from build123d import *

# Parameters (mm, degrees)
BOSS_EXTRU_1_DEPTH = 6


with BuildPart() as part:
    # Esquisse1 → Boss.-Extru.1 (new body)
    with BuildSketch(Plane.XY):
        with BuildLine():
            Line((-20.173501956, 71.960204906), (0, 185.65))
            Line((0, 185.65), (26, 157.518641754))
            Line((26, 157.518641754), (22.59550815, 72.124873891))
            ThreePointArc((22.59550815, 72.124873891), (25.386159845, 67.438342266), (30.801329033, 68.091992195))
            Line((30.801329033, 68.091992195), (119.333519738, 142.216150865))
            Line((119.333519738, 142.216150865), (121.168186735, 103.953802351))
            Line((121.168186735, 103.953802351), (63.670138745, 40.726746182))
            ThreePointArc((63.670138745, 40.726746182), (62.795457508, 35.34285834), (67.363875848, 32.362779578))
            Line((67.363875848, 32.362779578), (182.829559347, 32.237784184))
            Line((182.829559347, 32.237784184), (159.640432263, 1.747823511))
            Line((159.640432263, 1.747823511), (74.952803807, -9.727878693))
            ThreePointArc((74.952803807, -9.727878693), (70.822062709, -13.289941795), (72.406116488, -18.509337276))
            Line((72.406116488, -18.509337276), (160.777616213, -92.825))
            Line((160.777616213, -92.825), (123.415145329, -101.275981375))
            Line((123.415145329, -101.275981375), (51.16421896, -55.630721015))
            ThreePointArc((51.16421896, -55.630721015), (45.710237669, -55.704230463), (43.568730519, -60.72072951))
            Line((43.568730519, -60.72072951), (63.496039608, -174.453935049))
            Line((63.496039608, -174.453935049), (29.442540289, -156.911629019))
            Line((29.442540289, -156.911629019), (3.435327434, -75.503330707))
            ThreePointArc((3.435327434, -75.503330707), (-0.789915589, -72.053890614), (-5.654948672, -74.520217571))
            Line((-5.654948672, -74.520217571), (-63.496039608, -174.453935049))
            Line((-63.496039608, -174.453935049), (-78.30655657, -139.126581566))
            Line((-78.30655657, -139.126581566), (-45.900991977, -60.047092835))
            ThreePointArc((-45.900991977, -60.047092835), (-46.920458564, -54.688734557), (-52.232614532, -53.45086763))
            Line((-52.232614532, -53.45086763), (-160.777616213, -92.825))
            Line((-160.777616213, -92.825), (-149.415145329, -56.242660379))
            Line((-149.415145329, -56.242660379), (-73.75972711, -16.494152877))
            ThreePointArc((-73.75972711, -16.494152877), (-71.096397514, -11.734111803), (-74.370059552, -7.371262685))
            Line((-74.370059552, -7.371262685), (-182.829559347, 32.237784184))
            Line((-182.829559347, 32.237784184), (-150.610727024, 52.957826667))
            Line((-150.610727024, 52.957826667), (-67.10546618, 34.776584525))
            ThreePointArc((-67.10546618, 34.776584525), (-62.005541919, 36.711032274), (-61.708927176, 42.157437993))
            Line((-61.708927176, 42.157437993), (-119.333519738, 142.216150865))
            Line((-119.333519738, 142.216150865), (-81.333875693, 137.378758055))
            Line((-81.333875693, 137.378758055), (-29.05181183, 69.774971528))
            ThreePointArc((-29.05181183, 69.774971528), (-23.901604145, 67.978676352), (-20.173501956, 71.960204906))
        make_face()
        with BuildLine():
            Line((-7.5, 10.310795314), (-7.5, -10.310795314))
            ThreePointArc((-7.5, -10.310795314), (0, -12.75), (7.5, -10.310795314))
            Line((7.5, -10.310795314), (7.5, 10.310795314))
            ThreePointArc((7.5, 10.310795314), (0, 12.75), (-7.5, 10.310795314))
        make_face(mode=Mode.SUBTRACT)
    extrude(amount=BOSS_EXTRU_1_DEPTH)


solid = part.part
Geometry check sheet. Reference: the model listing, model coordinates, mm. A direction names the side the tool comes from. Round coordinates to 2 decimals unless told otherwise and drop trailing zeros. Loops run counter-clockwise (first coordinate to the right, second up) from the corner with the lowest first, then second, coordinate; pieces in that order, holes last.
Item 1: Cross-section at D-D on y = -32. Record the boundary of the cut face in (x, z), then the cut area to 3 significant figures.
Item 2: Thickness scan on line 1 (Y direction, x = 115, z = 4); line 2 (X direction, y = 108, z = 1.85); line 3 (X direction, y = 132, z = 2.55). Record the ranges inside material, lowest first.
Item 3: Access from +Z, -Z, +X, -X, +Y, -Y to the whole of each face (thin tool, end or side, straight path). Record for faces 1 (the flat face through (-112.12, -36.65, 2.96)), 2 (the flat face through (-55.56, 104.05, 2.96)), 3 (the flat face through (16.62, -116.78, 2.96)), 4 (the flat face through (-109.443, 43.994, 2.958)).
Item 4: Gauge pin test, flat ends, axial feed: pin 1 (1 mm diameter, centred on x = -105, z = 4, fed in from -Y); pin 2 (3 mm diameter, centred on x = -100.5, z = 5.5, fed in from +Y); pin 3 (1 mm diameter, centred on x = -29, z = 4.5, fed in from +Y). Record the tip position at first contact, or that the pin passes through.
Item 5: Cross-section at A-A on y = 80.5. Record the boundary of the cut face in (x, z).
Item 6: Mould release check, pull along X, two halves, no side actions. Record for faces 5 (the flat face through (142.36, -96.99, 2.96)), 6 (the flat face through (-155.176, -74.79, 2.958)), 7 (the flat face through (-62.33, -100.14, 2.96)), 8 (the flat face through (-13, -7, 0)): pulls with the +X half, pulls with the -X half, needs draft (parallel to the pull), parting line crosses it, or undercut.
Item 7: Cross-section at C-C on x = 110. Record the boundary of the cut face in (y, z), then the cut area to 3 significant figures.
Item 8: Cross-section at B-B on x = -134. Record the boundary of the cut face in (y, z).
Answer sheet:
1. outline: (-103.27, 0) - (88.45, 0) - (88.45, 6) - (-103.27, 6) - close
1. area: 1,150 mm2
2. line 1: y = -95.96 to -54.33, -4.3 to 32.31, 97.17 to 138.59
2. line 2: x = -99.63 to -58.61, -13.78 to 24.03, 78.47 to 120.97
2. line 3: x = -113.45 to -77.17, -9.52 to 24.98, 107.13 to 119.82
3. face 1: +Z, -Z, -X
3. face 2: +Z, -Z, +Y
3. face 3: +Z, -Z, -Y
3. face 4: +Z, -Z
4. pin 1: stops at y = -72.77
4. pin 2: stops at y = 140.01
4. pin 3: stops at y = 70.35
5. outline: (-83.79, 0) - (-37.35, 0) - (-37.35, 6) - (-83.79, 6) - close; (-18.66, 0) - (22.93, 0) - (22.93, 6) - (-18.66, 6) - close; (45.62, 0) - (99.84, 0) - (99.84, 6) - (45.62, 6) - close
6. face 5: pulls with the +X half
6. face 6: pulls with the -X half
6. face 7: undercut
6. face 8: needs draft
7. outline: (-92.8, 0) - (-50.12, 0) - (-50.12, 6) - (-92.8, 6) - close; (-4.98, 0) - (32.32, 0) - (32.32, 6) - (-4.98, 6) - close; (91.67, 0) - (134.4, 0) - (134.4, 6) - (91.67, 6) - close
7. area: 736 mm2
8. outline: (-83.11, 0) - (-48.14, 0) - (-48.14, 6) - (-83.11, 6) - close; (14.41, 0) - (49.34, 0) - (49.34, 6) - (14.41, 6) - close
